Part model, mm, in its own coordinate system. A direction names the side the tool comes from. Coordinates: 2 decimals unless noted, no trailing zeros. Loops run counter-clockwise (first coordinate to the right, second up) from the corner with the lowest first, then second, coordinate; pieces in that order, holes last. Notation, with made-up numbers: (-28, 16) - (-8, 16) arc R15 cw to (-8, 35) - close; hole circle Ø11 at (-32.5, -23). An arc over 180 degrees is marked (long way). Use a Markdown table: item, result. Add a question column.
1. Band-saw the part on D-D, the plane x = 13. Give the cut face in (y, z), plus the area to 3 significant figures.
2. Band-saw the part on B-B, the plane z = 15. Give the cut face in (x, y).
3. Band-saw the part on C-C, the plane z = 22.5. Give the cut face in (x, y).
4. Band-saw the part on A-A, the plane x = 21. Give the cut face in (y, z).
5. Drop flat-ended pins along their axis: pin 1 (6 mm diameter, centred on x = 32.5, z = 26, fed in from -Y); pin 2 (5 mm diameter, centred on y = -15, z = 17, fed in from +X). Give the stop position or say it passes through.
6. Wall check: probe 1 along Z at (x, y) = (32.5, -0.65); probe 2 along Y at (x, z) = (13.5, 2); probe 3 along Z at (x, y) = (9, -1). Give the ranges that are in metal, low to high. Write a range as [from, to].
7. 3-axis set-ups, long thin cutter, end or side, ignore diameter. For faces 1 (the flat face through (2, -40, 15)), 2 (the flat face through (2, -33, 13.25)), 3 (the flat face through (3, -17, 8)): which of +Z, -Z, +X, -X, +Y, -Y reach the whole face in a straight line?
8. Pull direction Z, two halves, no side cores. Call faces 4 (the flat face through (40, -1, 15)), 5 (the flat face through (2, -13, 13.25)), 6 (the flat face through (11, -2, 30)): pulls with the +Z half, pulls with the -Z half, needs draft (parallel to the pull), parting line crosses it, or undercut.
from build123d import *

# Parameters (mm, degrees)
BOSS_EXTRUDE1_DEPTH = 30
SKETCH2_R           = 11.05
SKETCH2_R_2         = 1.5
CUT_EXTRUDE1_DEPTH  = 4
CUT_EXTRUDE2_DEPTH  = 4


with BuildPart() as part:
    # Sketch1 → Boss-Extrude1 (new body)
    with BuildSketch(Plane.XY):
        Polygon((0, 0), (40, 0), (40, -3), (3, -3), (3, -40), (0, -40), (0, -3), align=None)
    extrude(amount=BOSS_EXTRUDE1_DEPTH)

    # Sketch2 → Cut-Extrude1 (cut, through all)
    with BuildSketch(Plane.XZ.offset(3)):
        with Locations((21, 15)):
            Circle(SKETCH2_R)
        with Locations((32.502183488, 26.5)):
            Circle(SKETCH2_R_2)
        with Locations((32.5, 3.497816512)):
            Circle(SKETCH2_R_2)
        with Locations((9.497816512, 3.5)):
            Circle(SKETCH2_R_2)
        with Locations((9.5, 26.502183488)):
            Circle(SKETCH2_R_2)
    extrude(amount=-CUT_EXTRUDE1_DEPTH, mode=Mode.SUBTRACT)

    # Sketch3 → Cut-Extrude2 (cut, through all)
    with BuildSketch(Plane(origin=(3, 0, 0), x_dir=(0, 0, -1), z_dir=(1, 0, 0))):
        with BuildLine():
            Line((-26, -21.27), (-23.389421911, -21.27))
            ThreePointArc((-23.389421911, -21.27), (-21.059905115, -16.960094885), (-16.75, -14.630578089))
            Line((-16.75, -14.630578089), (-16.75, -12.02))
            ThreePointArc((-16.75, -12.02), (-15, -10.27), (-13.25, -12.02))
            Line((-13.25, -12.02), (-13.25, -14.630578089))
            ThreePointArc((-13.25, -14.630578089), (-8.940094885, -16.960094885), (-6.610578089, -21.27))
            Line((-6.610578089, -21.27), (-4, -21.27))
            ThreePointArc((-4, -21.27), (-2.25, -23.02), (-4, -24.77))
            Line((-4, -24.77), (-6.610578089, -24.77))
            ThreePointArc((-6.610578089, -24.77), (-8.940094885, -29.079905115), (-13.25, -31.409421911))
            Line((-13.25, -31.409421911), (-13.25, -34.02))
            ThreePointArc((-13.25, -34.02), (-15, -35.77), (-16.75, -34.02))
            Line((-16.75, -34.02), (-16.75, -31.409421911))
            ThreePointArc((-16.75, -31.409421911), (-21.059905115, -29.079905115), (-23.389421911, -24.77))
            Line((-23.389421911, -24.77), (-26, -24.77))
            ThreePointArc((-26, -24.77), (-27.75, -23.02), (-26, -21.27))
        make_face()
    extrude(amount=-CUT_EXTRUDE2_DEPTH, mode=Mode.SUBTRACT)


solid = part.part
Geometry check:
| question | item | result |
|---|---|---|
| 1 | outline | (-3, 0) - (0, 0) - (0, 7.38) - (-3, 7.38) - close; (-3, 22.62) - (0, 22.62) - (0, 30) - (-3, 30) - close |
| 1 | area | 44.3 mm^2 |
| 2 | outline | (0, -40) - (3, -40) - (3, -35.77) - (0, -35.77) - close; (0, -10.27) - (3, -10.27) - (3, -3) - (9.95, -3) - (9.95, 0) - (0, 0) - close; (32.05, -3) - (40, -3) - (40, 0) - (32.05, 0) - close |
| 3 | outline | (0, -40) - (3, -40) - (3, -27.17) - (0, -27.17) - close; (0, -18.87) - (3, -18.87) - (3, -3) - (12.89, -3) - (12.89, 0) - (0, 0) - close; (29.11, -3) - (40, -3) - (40, 0) - (29.11, 0) - close |
| 4 | outline | (-3, 0) - (0, 0) - (0, 3.95) - (-3, 3.95) - close; (-3, 26.05) - (0, 26.05) - (0, 30) - (-3, 30) - close |
| 5 | pin 1 | stops at y = -3 |
| 5 | pin 2 | stops at x = 3 |
| 6 | probe 1 | z = [0, 2], [5, 25], [28, 30] |
| 6 | probe 2 | y = [-3, 0] |
| 6 | probe 3 | z = [0, 2.09], [4.91, 25.09], [27.92, 30] |
| 7 | face 1 | +Z, -Z, +X, -X, -Y |
| 7 | face 2 | +X, -X |
| 7 | face 3 | +Z, -Z, +X, -Y |
| 8 | face 4 | needs draft |
| 8 | face 5 | undercut |
| 8 | face 6 | pulls with the +Z half |
